The drawing under review shows one solid part. Ordinate dimensions are in mm from its lowest x, y, z. Round coordinates to 2 decimals unless told otherwise and drop trailing zeros. Order: outer loops, then holes, each group sorted by start corner. A loop starts at its lowest first (then second) coordinate and runs counter-clockwise, first axis right, second up.
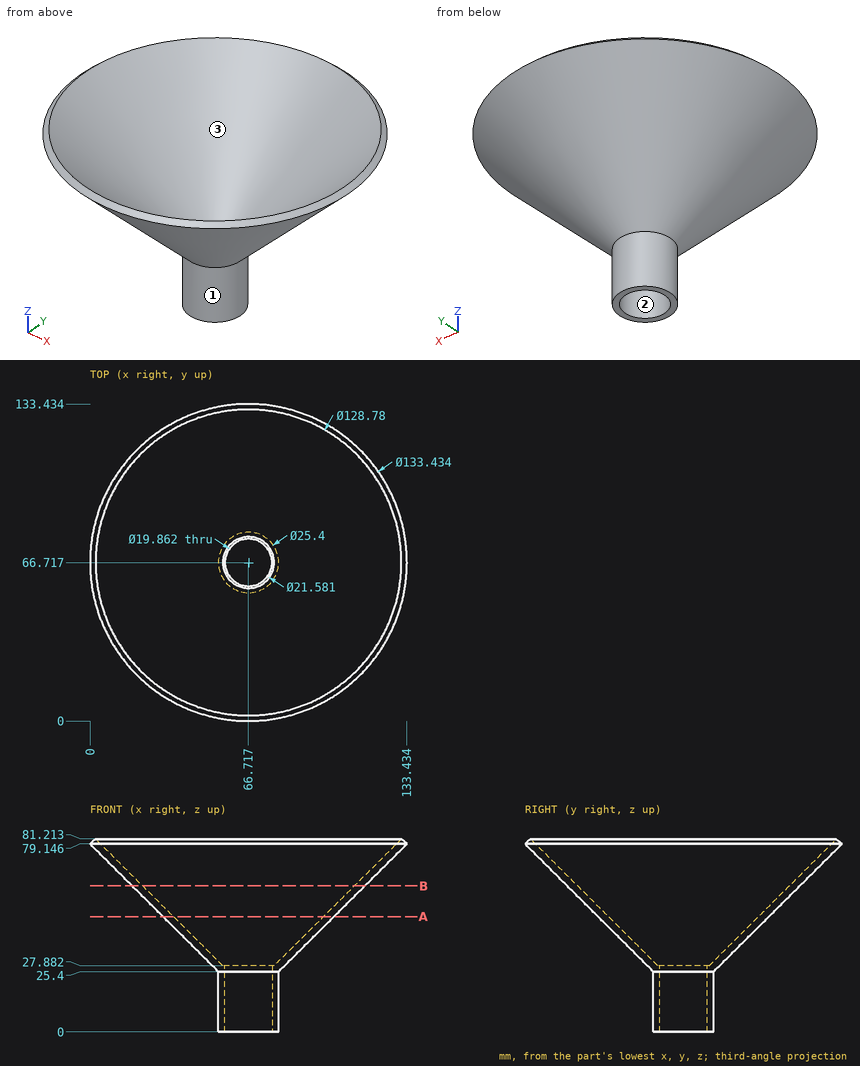
(1) Clearance check with flat-ended pins moving along their axes: P1, Ø4, axis at x = 71, z = 70.5, coming from the +Y side; P2, Ø8, axis at x = 59.5, y = 110, coming from the +Z side (1 decimal); P3, Ø10, axis at x = 94.5, z = 51.5, coming from the +Y side. State where each tip first meets the part, or that it passes through.
(2) We need section B-B (z = 61.5). Give the boundary of the cut face in (x, y) (1 decimal).
(3) The part is to be moulded in two halves that separate along Y. For the marked faces 1, 2 and 3, say which applies: pulls with the +Y half, pulls with the -Y half, needs draft (parallel to the pull), parting line crosses it, or undercut.
(4) We need section A-A (z = 48.5). Give the boundary of the cut face in (x, y) (1 decimal).
(5) To check wall thickness, follow L1, parallel to Y at x = 37.5, z = 63 (1 decimal); L2, parallel to Y at x = 101, z = 72.5 (1 decimal); L3, parallel to X at y = 58.5, z = 74.5 (1 decimal). State the ranges of each line that lie inside material, in increasing order.
Verdict:
1. P1: stops at y = 126.61
1. P2: stops at z = 64.8
1. P3: stops at y = 101.85
2. outline: circle Ø98 at (66.7, 66.7); hole circle Ø89.2 at (66.7, 66.7)
3. face 1: parting line crosses it
3. face 2: undercut
3. face 3: undercut
4. outline: circle Ø71.8 at (66.7, 66.7); hole circle Ø63 at (66.7, 66.7)
5. L1: y = 25.5 to 31.1, 102.4 to 107.9
5. L2: y = 17.4 to 22.9, 110.5 to 116
5. L3: x = 5.2 to 9.7, 123.8 to 128.2
